Geometry check sheet. Reference: the model listing, model coordinates, mm. A direction names the side the tool comes from. Coordinates: 2 decimals unless noted, no trailing zeros. Order: outer loops, then holes, each group sorted by start corner. A loop starts at its lowest first (then second) coordinate and runs counter-clockwise, first axis right, second up. Notation, with made-up numbers: M 1,42 L 13,42 A19 cw 13,65 Z; hole C -18,-39 d4. An arc over 180 degrees is marked long. Use CSV: the item, a comma, the result in double quotes. Start each with the question number.
```python
from build123d import *

# Parameters (mm, degrees)
SKETCH1_W           = 114.3
SKETCH1_H           = 177.8
BOSS_EXTRUDE1_DEPTH = 3.175
SKETCH2_R           = 2.54
CUT_EXTRUDE1_DEPTH  = 3.175
FILLET1_R           = 12.7
CUT_EXTRUDE2_DEPTH  = 106.732743864
FILLET2_R           = 2.54


with BuildPart() as part:
    # Sketch1 → Boss-Extrude1 (new body)
    with BuildSketch(Plane(origin=(0, 0, 0), x_dir=(1, 0, 0), z_dir=(0, 1, 0))):
        Rectangle(SKETCH1_W, SKETCH1_H)
    extrude(amount=BOSS_EXTRUDE1_DEPTH)

    # Sketch2 → Cut-Extrude1 (cut)
    with BuildSketch(Plane(origin=(0, 3.175, 0), x_dir=(1, 0, 0), z_dir=(0, 1, 0))):
        with Locations(Location((-44.45, 76.2, 0), (0, 0, 270))):
            Circle(SKETCH2_R)
        with Locations(Location((-44.45, 54.428571429, 0), (0, 0, 270))):
            Circle(SKETCH2_R)
        with Locations(Location((-44.45, 32.657142857, 0), (0, 0, 270))):
            Circle(SKETCH2_R)
        with Locations(Location((-44.45, 10.885714286, 0), (0, 0, 270))):
            Circle(SKETCH2_R)
        with Locations(Location((-44.45, -10.885714286, 0), (0, 0, 270))):
            Circle(SKETCH2_R)
        with Locations(Location((-44.45, -32.657142857, 0), (0, 0, 270))):
            Circle(SKETCH2_R)
        with Locations(Location((-44.45, -54.428571429, 0), (0, 0, 270))):
            Circle(SKETCH2_R)
        with Locations(Location((-44.45, -76.2, 0), (0, 0, 270))):
            Circle(SKETCH2_R)
        with Locations(Location((44.45, -76.2, 0), (0, 0, 90))):
            Circle(SKETCH2_R)
        with Locations(Location((44.45, -54.428571429, 0), (0, 0, 90))):
            Circle(SKETCH2_R)
        with Locations(Location((44.45, -32.657142857, 0), (0, 0, 90))):
            Circle(SKETCH2_R)
        with Locations(Location((44.45, -10.885714286, 0), (0, 0, 90))):
            Circle(SKETCH2_R)
        with Locations(Location((44.45, 10.885714286, 0), (0, 0, 90))):
            Circle(SKETCH2_R)
        with Locations(Location((44.45, 32.657142857, 0), (0, 0, 90))):
            Circle(SKETCH2_R)
        with Locations(Location((44.45, 54.428571429, 0), (0, 0, 90))):
            Circle(SKETCH2_R)
        with Locations(Location((44.45, 76.2, 0), (0, 0, 90))):
            Circle(SKETCH2_R)
    extrude(amount=-CUT_EXTRUDE1_DEPTH, mode=Mode.SUBTRACT)

    # Fillet1
    fillet1_edges = [part.edges().sort_by_distance(p)[0] for p in [
        (57.15, 1.5875, 88.9),
        (-57.15, 1.5875, 88.9),
        (-57.15, 1.5875, -88.9),
        (57.15, 1.5875, -88.9),
    ]]
    fillet(fillet1_edges, radius=FILLET1_R)

    # Sketch3 → Cut-Extrude2 (cut, through all)
    with BuildSketch(Plane(origin=(0, 3.175, 0), x_dir=(1, 0, 0), z_dir=(0, 1, 0))):
        Polygon((27.6225, -76.2), (-27.6225, -76.2), (0, -9.906), align=None)
        Polygon((31.75, -66.294), (31.75, 66.294), (4.1275, 0), align=None)
        Polygon((27.6225, 76.2), (-27.6225, 76.2), (0, 9.906), align=None)
        Polygon((-31.75, -66.294), (-31.75, 66.294), (-4.1275, 0), align=None)
    extrude(amount=-CUT_EXTRUDE2_DEPTH, mode=Mode.SUBTRACT)

    # Fillet2
    fillet2_edges = [part.edges().sort_by_distance(p)[0] for p in [
        (31.75, 1.5875, 66.294),
        (4.1275, 1.5875, 0),
        (31.75, 1.5875, -66.294),
        (-4.1275, 1.5875, 0),
        (-31.75, 1.5875, 66.294),
        (-31.75, 1.5875, -66.294),
        (0, 1.5875, -9.906),
        (-27.6225, 1.5875, -76.2),
        (27.6225, 1.5875, -76.2),
        (0, 1.5875, 9.906),
        (27.6225, 1.5875, 76.2),
        (-27.6225, 1.5875, 76.2),
    ]]
    fillet(fillet2_edges, radius=FILLET2_R)


solid = part.part
```
1) Gauge pin test, flat ends, axial feed: P1, Ø3, axis at x = -44.45, z = -32.66, coming from the +Y side; P2, Ø6, axis at x = 44.45, z = 54.43, coming from the -Y side. Record the tip position at first contact, or that the pin passes through.
2) Section check C-C on z = 61. Record the boundary of the cut face in (x, y) (3 decimals), then the cut area to 3 significant figures.
3) Material ranges on line 1 along Z through (x, y) = (-25.5, 0.4); line 2 along X through (y, z) = (1.8, 17); line 3 along Z through (x, y) = (-1.5, 0.6), recorded low to high.
4) Section check B-B on x = 21.5. Record the boundary of the cut face in (y, z) (3 decimals).
5) Set-up check for faces 1 (the face through (-15.856, 1.61, -28.149)), 2 (the face through (-1, 2, -88.9)): record each of +Z, -Z, +X, -X, +Y, -Y from which the full face is reachable in a straight line by a thin tool's end or side.
6) Section check A-A on z = -33. State how many separate pieces and enclosed holes the cut face has, then the cut area to 3 significant figures.
Results are:
1,P1,"passes through"
1,P2,"stops at y = 0"
2,outline,"M -57.15,0 L -21.289,0 L -21.289,3.175 L -57.15,3.175 Z; M 21.289,0 L 57.15,0 L 57.15,3.175 L 21.289,3.175 Z"
2,area,"228 mm²"
3,line 1,"z = -88.9 to -75.56, -71.11 to -51.29, 51.29 to 71.11, 75.56 to 88.9"
3,line 2,"x = -57.15 to -31.75, -11.21 to -2.96, 2.96 to 11.21, 31.75 to 57.15"
3,line 3,"z = -88.9 to -76.2, -14.46 to 14.46, 76.2 to 88.9"
4,outline,"M 0,-88.9 L 3.175,-88.9 L 3.175,-76.2 L 0,-76.2 Z; M 0,-61.506 L 3.175,-61.506 L 3.175,-41.694 L 0,-41.694 Z; M 0,41.694 L 3.175,41.694 L 3.175,61.506 L 0,61.506 Z; M 0,76.2 L 3.175,76.2 L 3.175,88.9 L 0,88.9 Z"
5,face 1,"+Y, -Y"
5,face 2,"-Z, +X, -X, +Y, -Y"
6,separate pieces,"6"
6,enclosed holes,"0"
6,area,"182 mm²"
